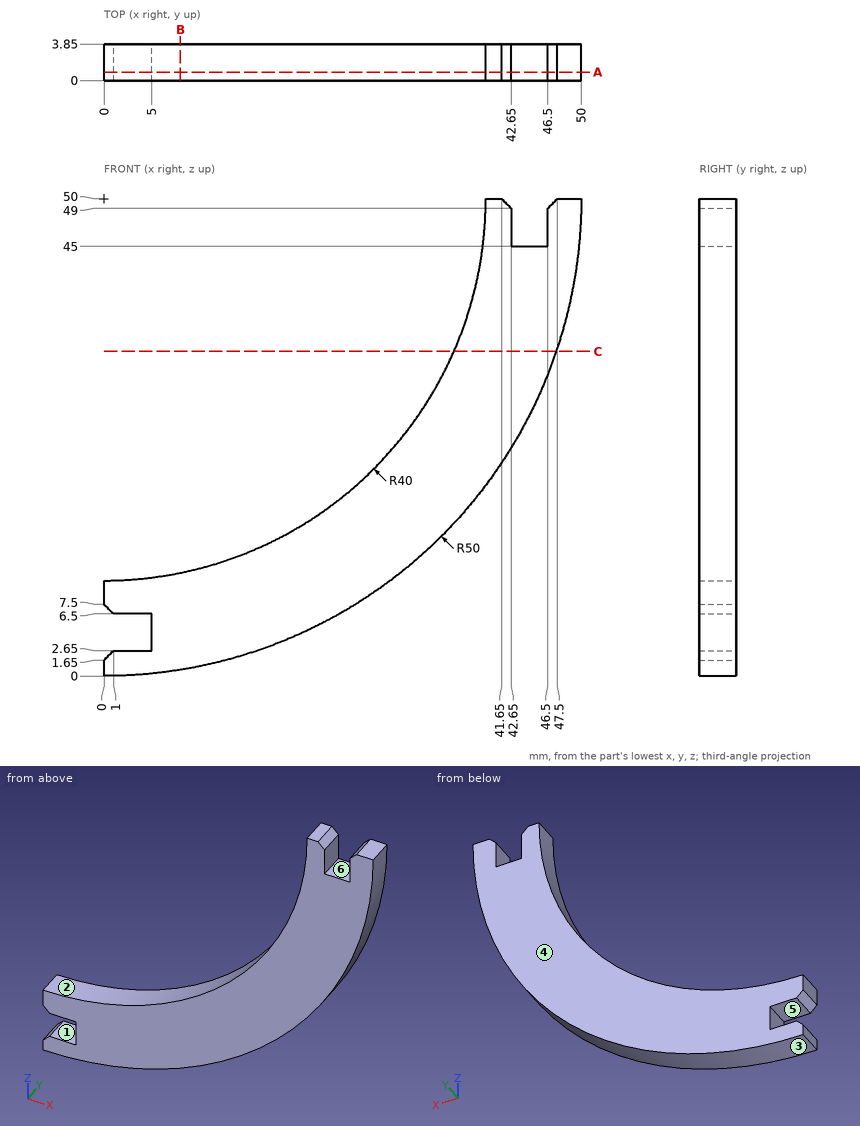
The figure shows three views and two pictorial views of one solid part (mm, origin at its lowest corner). Answer the questions. A direction names the side the tool comes from. Round coordinates to 2 decimals unless told otherwise and drop trailing zeros. Order: outer loops, then holes, each group sorted by start corner. A loop starts at its lowest first (then second) coordinate and runs counter-clockwise, first axis right, second up. Notation, with made-up numbers: M 54.5,63.25 L 77.5,63.25 A26 ccw 77.5,87.25 Z; hole C -40,-29.75 d6. An arc over 180 degrees is marked long. Answer in a Markdown table with one row per item. Add a question column.
1) The part is cut by section B-B on x = 8. Determine the outline of the cut face in (y, z).
2) Flat-ended cylindrical pins translate along their axes: pin 1 Ø2 at (x, y) = (11.5, 1) entering from -Z; pin 2 Ø1.5 at (x, y) = (35.5, 2.5) entering from +Z. Find the tip coordinate at first contact, or state that the pin passes through.
3) Which of the six approach directions +Z, -Z, +X, -X, +Y, -Y give full straight-line access (tool end or side, diameter ignored) to the marked faces 4, 5 and 6?
4) The part is cut by section A-A on y = 0.9. Determine the outline of the cut face in (x, z).
5) The part is cut by section C-C on z = 34. Determine the outline of the cut face in (x, y), plus the area to 3 significant figures.
6) Determine the mould class of the marked faces 1, 2 and 3 for opening direction Z: pulls with the +Z half, pulls with the -Z half, needs draft (parallel to the pull), parting line crosses it, or undercut.
7) Consider line 1 along Z through (x, y) = (2, 3.4); line 2 along Z through (x, y) = (3, 3.75); line 3 along Z through (x, y) = (16.5, 2.5). Determine where each line is inside the solid, lowest interval first. Write a range as from..to.
Findings below:
| question | item | result |
|---|---|---|
| 1 | outline | M 0,0.64 L 3.85,0.64 L 3.85,10.81 L 0,10.81 Z |
| 2 | pin 1 | stops at z = 1.11 |
| 2 | pin 2 | stops at z = 33.09 |
| 3 | face 4 | +Z, -Z, +X, -X, +Y |
| 3 | face 5 | -X, +Y, -Y |
| 3 | face 6 | +Z, +Y, -Y |
| 4 | outline | M 0,0 A50 ccw 50,50 L 47.5,50 L 46.5,49 L 46.5,45 L 42.65,45 L 42.65,49 L 41.65,50 L 40,50 A40 cw 0,10 L 0,7.5 L 1,6.5 L 5,6.5 L 5,2.65 L 1,2.65 L 0,1.65 Z |
| 5 | outline | M 36.66,0 L 47.37,0 L 47.37,3.85 L 36.66,3.85 Z |
| 5 | area | 41.2 mm² |
| 6 | face 1 | undercut |
| 6 | face 2 | pulls with the +Z half |
| 6 | face 3 | pulls with the -Z half |
| 7 | line 1 | z = 0.04..2.65, 6.5..10.05 |
| 7 | line 2 | z = 0.09..2.65, 6.5..10.11 |
| 7 | line 3 | z = 2.8..13.56 |
